```python
from build123d import *

# Parameters (mm, degrees)
SKETCH1_W           = 20
SKETCH1_H           = 30
BOSS_EXTRUDE1_DEPTH = 15
SKETCH2_W           = 6.2
SKETCH2_H           = 6.2
CUT_EXTRUDE1_DEPTH  = 3.25
FILLET1_R           = 5
SKETCH4_W           = 6.2
SKETCH4_H           = 6.2
CUT_EXTRUDE2_DEPTH  = 68
SKETCH6_W           = 5
SKETCH6_H           = 1
BOSS_EXTRUDE3_DEPTH = 6.2
SKETCH7_R           = 0.75
CUT_EXTRUDE3_DEPTH  = 37


with BuildPart() as part:
    # Sketch1 → Boss-Extrude1 (new body)
    with BuildSketch(Plane.XY):
        with Locations((-36.265495527, 120.408164147)):
            Rectangle(SKETCH1_W, SKETCH1_H)
    extrude(amount=BOSS_EXTRUDE1_DEPTH)

    # Sketch2 → Cut-Extrude1 (cut)
    with BuildSketch(Plane(origin=(0, 105.408164147, 0), x_dir=(-1, 0, 0), z_dir=(0, -1, 0))):
        with Locations((36.265495527, -7.5)):
            Rectangle(SKETCH2_W, SKETCH2_H)
    extrude(amount=-CUT_EXTRUDE1_DEPTH, mode=Mode.SUBTRACT)

    # Fillet1
    fillet1_edges = [part.edges().sort_by_distance(p)[0] for p in [
        (-46.265495527, 120.408164147, 15),
        (-26.265495527, 120.408164147, 15),
        (-46.265495527, 120.408164147, 0),
        (-36.265495527, 135.408164147, 0),
        (-26.265495527, 120.408164147, 0),
        (-36.265495527, 135.408164147, 15),
        (-46.265495527, 135.408164147, 7.5),
        (-26.265495527, 135.408164147, 7.5),
    ]]
    fillet(fillet1_edges, radius=FILLET1_R)

    # Sketch4 → Cut-Extrude2 (cut)
    with BuildSketch(Plane.XZ.offset(-108.658164147)):
        with Locations((-36.265495527, 7.5)):
            Rectangle(SKETCH4_W, SKETCH4_H)
    extrude(amount=-CUT_EXTRUDE2_DEPTH, mode=Mode.SUBTRACT)

    # Sketch6 → Boss-Extrude3 (add)
    with BuildSketch(Plane(origin=(-39.365495527, 0, 0), x_dir=(0, 0, -1), z_dir=(1, 0, 0))):
        with Locations((-7.5, 134.949726458)):
            Rectangle(SKETCH6_W, SKETCH6_H)
    extrude(amount=BOSS_EXTRUDE3_DEPTH)

    # Sketch7 → Cut-Extrude3 (cut)
    with BuildSketch(Plane.XZ.offset(-105.408164147)):
        with Locations(Location((-36.265495527, 12.8, 0), (0, 0, 270))):
            Circle(SKETCH7_R)
    extrude(amount=-CUT_EXTRUDE3_DEPTH, mode=Mode.SUBTRACT)


solid = part.part
```
Input: part model. Units: mm. Frame: model coordinates. A direction names the side the tool comes from. Round coordinates to 2 decimals unless told otherwise and drop trailing zeros. Write each loop counter-clockwise with the first axis right and the second up, starting at its lowest first coordinate (ties: lowest second). Pieces come first, ordered by that corner, then holes. Notation, with made-up numbers: (-22.75, 78.5) -> (25.25, 78.5) arc R22 ccw to (25.25, 115.5) -> close; hole circle Ø8 at (6.5, 78). An arc over 180 degrees is marked (long way). Answer as CSV lines item,"result".
1. Section A-A (y = 121). Return the cut outline in (x, z), plus the area to 3 significant figures.
Geometry says:
outline,"(-46.27, 5) arc R5 ccw to (-41.27, 0) -> (-31.27, 0) arc R5 ccw to (-26.27, 5) -> (-26.27, 10) arc R5 ccw to (-31.27, 15) -> (-41.27, 15) arc R5 ccw to (-46.27, 10) -> close; hole (-39.37, 4.4) -> (-33.17, 4.4) -> (-33.17, 10.6) -> (-39.37, 10.6) -> close; hole circle Ø1.5 at (-36.27, 12.8)"
area,"238 mm^2"
2. Reachability of faces 4 (the flat face through (-39.365, 120, 8)), 5 (the flat face through (-36, 120, 4.4)), 6 (the flat face through (-32, 135.408, 7)) from +Z, -Z, +X, -X, +Y, -Y: full face, straight path, thin tool, end or side. Return the list, or none.
Geometry says:
face 4,"-Y"
face 5,"+Y, -Y"
face 6,"+Z, -Z, +X, +Y"
3. Ray query, L1, parallel to X at y = 125, z = 5.5; L2, parallel to Z at x = -36, y = 130; L3, parallel to Z at x = -39.25, y = 127. Return the intervals inside material, ascending. Write a range as [from, to].
Geometry says:
L1,"x = [-46.27, -39.37], [-33.17, -26.27]"
L2,"z = [0, 4.4], [10.6, 12.1], [13.5, 15]"
L3,"z = [0, 4.4], [10.6, 15]"
4. Mould query, pull axis X, two halves, no side actions, for faces 1 (the flat face through (-36, 135, 10)), 2 (the flat face through (-26.265, 118, 7)), 3 (the flat face through (-36, 105.408, 4)). Classes: +X half, -X half, draft (parallel to the pull), parting line (faces both ways), or undercut.
Geometry says:
face 1,"undercut"
face 2,"+X half"
face 3,"draft"
5. Section D-D (z = 12.8). Return the cut outline in (x, y), plus the area to 3 significant figures.
Geometry says:
outline,"(-45.41, 105.41) -> (-37.02, 105.41) -> (-37.02, 134.55) -> (-41.27, 134.55) arc R4.14 ccw to (-45.41, 130.41) -> close; (-35.52, 105.41) -> (-27.12, 105.41) -> (-27.12, 130.41) arc R4.14 ccw to (-31.27, 134.55) -> (-35.52, 134.55) -> close"
area,"482 mm^2"
6. Contact query for flat-ended pins moving along their axis: P1, Ø5, axis at y = 119.5, z = 13, coming from the +X side; P2, Ø0.9, axis at x = -40, z = 7.5, coming from the +Y side; P3, Ø0.8, axis at x = -35, y = 135, coming from the -Z side; P4, Ø1.2, axis at x = -36.27, z = 12.8, coming from the +Y side (3 decimals). Output: stop coordinate, or through.
Geometry says:
P1,"stops at x = -26.29"
P2,"stops at y = 135.41"
P3,"stops at z = 2.27"
P4,"passes through"
7. Section B-B (z = 8.25). Return the cut outline in (x, y), plus the area to 3 significant figures.
Geometry says:
outline,"(-46.27, 105.41) -> (-39.37, 105.41) -> (-39.37, 134.45) -> (-33.17, 134.45) -> (-33.17, 105.41) -> (-26.27, 105.41) -> (-26.27, 130.41) arc R5 ccw to (-31.27, 135.41) -> (-33.17, 135.41) -> (-33.17, 135.45) -> (-39.37, 135.45) -> (-39.37, 135.41) -> (-41.27, 135.41) arc R5 ccw to (-46.27, 130.41) -> close"
area,"409 mm^2"
8. Section C-C (x = -40.25). Return the cut outline in (y, z).
Geometry says:
outline,"(105.41, 0) -> (130.41, 0) arc R5 ccw to (135.41, 5) -> (135.41, 10) arc R5 ccw to (130.41, 15) -> (105.41, 15) -> close"
